Design review of the part built by this model. Coordinates are the model's own, in mm. Round coordinates to 2 decimals unless told otherwise and drop trailing zeros. Write each loop counter-clockwise with the first axis right and the second up, starting at its lowest first coordinate (ties: lowest second). Pieces come first, ordered by that corner, then holes. Notation, with made-up numbers: (57.5, 57) -> (116.5, 57) arc R14 cw to (116.5, 73) -> close; hole circle Ø9 at (84, 26). An arc over 180 degrees is marked (long way). Write item = value, one per line. Start each with the question number.
Item 1: To check wall thickness, follow L1, parallel to Z at x = 0, y = -7.5; L2, parallel to Z at x = -9.25, y = -3; L3, parallel to X at y = -2.25, z = 32.5. State the ranges of each line that lie inside material, in increasing order.
Item 2: Mouldability with a two-part tool opening along X and no side actions: class faces 1 (the flat face through (25, -5, -1)), 2 (the cylindrical face through (8.06, -5.07, 8.34)), 3 (the flat face through (0, -5, 45)) as released by +X, released by -X, zero draft, split by the parting line, or undercut.
Item 3: Add section B-B, the plane z = 28.5. State the section outline as (x, y) points.
Item 4: Add section A-A, the plane x = 0. State the section outline as (y, z) points, then the cut area to 3 significant figures.
from build123d import *

# Parameters (mm, degrees)
F0_W     = 50
F0_H     = 90
F1_DEPTH = 10
F2_R     = 4
F2_R_2   = 1.5
F3_DEPTH = 25


with BuildPart() as f1:
    # F0 (on Front) → F1 (new body)
    with BuildSketch(Plane.XZ):
        Rectangle(F0_W, F0_H)
    extrude(amount=F1_DEPTH)

    # F2 (on face) → F3 (cut)
    with BuildSketch(Plane.XZ.offset(10)):
        with Locations((0, 30)):
            Circle(F2_R)
        with Locations((9.25, 9.25)):
            Circle(F2_R_2)
        with Locations((-9.25, 9.25)):
            Circle(F2_R_2)
    extrude(amount=-F3_DEPTH, mode=Mode.SUBTRACT)


solid = f1.part
Result set:
q1.L1 = -45 to 26, 34 to 45
q1.L2 = -45 to 7.75, 10.75 to 45
q1.L3 = -25 to -3.12, 3.12 to 25
q2.face_1 = released by +X
q2.face_2 = undercut
q2.face_3 = zero draft
q3.outline = (-25, -10) -> (-3.71, -10) -> (-3.71, 0) -> (-25, 0) -> close; (3.71, -10) -> (25, -10) -> (25, 0) -> (3.71, 0) -> close
q4.outline = (-10, -45) -> (0, -45) -> (0, 26) -> (-10, 26) -> close; (-10, 34) -> (0, 34) -> (0, 45) -> (-10, 45) -> close
q4.area = 820 mm²
